Can you work these out from the model? Positions are in its coordinate system, mm. A direction names the side the tool comes from. Give positions to 0.01 mm unless a question says otherwise; leave off trailing zeros. Write each loop counter-clockwise with the first axis right and the second up, starting at its lowest first coordinate (ties: lowest second). Pieces come first, ordered by that corner, then holes.
from build123d import *

# Parameters (mm, degrees)
SKETCH1_W            = 52
SKETCH1_H            = 40
SKETCH1_R            = 2.75
BOSS_EXTRUDE10_DEPTH = 5
SKETCH1_21_R         = 2.75
BOSS_EXTRUDE13_DEPTH = 5
SKETCH1_22_R         = 2.12
CUT_EXTRUDE4_DEPTH   = 7
CHAMFER1_SIZE        = 1
SKETCH1_23_R         = 2.75
BOSS_EXTRUDE14_DEPTH = 5
SKETCH1_24_R         = 2.12
CUT_EXTRUDE6_DEPTH   = 5
SKETCH1_25_R         = 2.75
BOSS_EXTRUDE15_DEPTH = 5
SKETCH1_26_R         = 2.12
CUT_EXTRUDE7_DEPTH   = 18
SKETCH1_29_R         = 2.75
BOSS_EXTRUDE17_DEPTH = 5
SKETCH1_30_R         = 2.12
CUT_EXTRUDE9_DEPTH   = 14
CHAMFER3_SIZE        = 1
CHAMFER4_SIZE        = 1
CHAMFER5_SIZE        = 1
SKETCH5_W            = 104
SKETCH5_H            = 97.258090947
BOSS_EXTRUDE19_DEPTH = 8


with BuildPart() as part:
    # Sketch1 → Boss-Extrude10 (new body)
    with BuildSketch(Plane(origin=(0, 0, 0), x_dir=(1, 0, 0), z_dir=(0, 1, 0))):
        Rectangle(SKETCH1_W, SKETCH1_H)
        with Locations(Location((-20, 4, 0), (0, 0, 270))):
            Circle(SKETCH1_R, mode=Mode.SUBTRACT)
        with Locations(Location((20, 4, 0), (0, 0, 270))):
            Circle(SKETCH1_R, mode=Mode.SUBTRACT)
        with Locations(Location((-20, -12, 0), (0, 0, 270))):
            Circle(SKETCH1_R, mode=Mode.SUBTRACT)
        with Locations(Location((20, -12, 0), (0, 0, 270))):
            Circle(SKETCH1_R, mode=Mode.SUBTRACT)
    extrude(amount=BOSS_EXTRUDE10_DEPTH)

    # Sketch1_21 → Boss-Extrude13 (add)
    with BuildSketch(Plane(origin=(0, 0, 0), x_dir=(1, 0, 0), z_dir=(0, 1, 0))):
        with Locations((20, 4)):
            Circle(SKETCH1_21_R)
    extrude(amount=BOSS_EXTRUDE13_DEPTH)

    # Sketch1_22 → Cut-Extrude4 (cut)
    with BuildSketch(Plane(origin=(0, 0, 0), x_dir=(1, 0, 0), z_dir=(0, 1, 0))):
        with Locations(Location((20, 4, 0), (0, 0, 90))):
            Circle(SKETCH1_22_R)
    extrude(amount=CUT_EXTRUDE4_DEPTH, mode=Mode.SUBTRACT)

    # Chamfer1
    chamfer1_edges = [part.edges().sort_by_distance(p)[0] for p in [
        (20, 5, -1.88),
    ]]
    chamfer(chamfer1_edges, length=CHAMFER1_SIZE)

    # Sketch1_23 → Boss-Extrude14 (add)
    with BuildSketch(Plane(origin=(0, 0, 0), x_dir=(1, 0, 0), z_dir=(0, 1, 0))):
        with Locations((20, -12)):
            Circle(SKETCH1_23_R)
    extrude(amount=BOSS_EXTRUDE14_DEPTH)

    # Sketch1_24 → Cut-Extrude6 (cut)
    with BuildSketch(Plane(origin=(0, 0, 0), x_dir=(1, 0, 0), z_dir=(0, 1, 0))):
        with Locations(Location((20, -12, 0), (0, 0, 90))):
            Circle(SKETCH1_24_R)
    extrude(amount=CUT_EXTRUDE6_DEPTH, mode=Mode.SUBTRACT)

    # Sketch1_25 → Boss-Extrude15 (add)
    with BuildSketch(Plane(origin=(0, 0, 0), x_dir=(1, 0, 0), z_dir=(0, 1, 0))):
        with Locations((-20, -12)):
            Circle(SKETCH1_25_R)
    extrude(amount=BOSS_EXTRUDE15_DEPTH)

    # Sketch1_26 → Cut-Extrude7 (cut)
    with BuildSketch(Plane(origin=(0, 0, 0), x_dir=(1, 0, 0), z_dir=(0, 1, 0))):
        with Locations(Location((-20, -12, 0), (0, 0, 270))):
            Circle(SKETCH1_26_R)
    extrude(amount=CUT_EXTRUDE7_DEPTH, mode=Mode.SUBTRACT)

    # Sketch1_29 → Boss-Extrude17 (add)
    with BuildSketch(Plane(origin=(0, 0, 0), x_dir=(1, 0, 0), z_dir=(0, 1, 0))):
        with Locations((-20, 4)):
            Circle(SKETCH1_29_R)
    extrude(amount=BOSS_EXTRUDE17_DEPTH)

    # Sketch1_30 → Cut-Extrude9 (cut)
    with BuildSketch(Plane(origin=(0, 0, 0), x_dir=(1, 0, 0), z_dir=(0, 1, 0))):
        with Locations(Location((-20, 4, 0), (0, 0, 270))):
            Circle(SKETCH1_30_R)
    extrude(amount=CUT_EXTRUDE9_DEPTH, mode=Mode.SUBTRACT)

    # Chamfer3
    chamfer3_edges = [part.edges().sort_by_distance(p)[0] for p in [
        (-20, 5, -6.12),
    ]]
    chamfer(chamfer3_edges, length=CHAMFER3_SIZE)

    # Chamfer4
    chamfer4_edges = [part.edges().sort_by_distance(p)[0] for p in [
        (-20, 5, 9.88),
    ]]
    chamfer(chamfer4_edges, length=CHAMFER4_SIZE)

    # Chamfer5
    chamfer5_edges = [part.edges().sort_by_distance(p)[0] for p in [
        (20, 5, 14.12),
    ]]
    chamfer(chamfer5_edges, length=CHAMFER5_SIZE)

    # Sketch5 → Boss-Extrude19 (add)
    with BuildSketch(Plane(origin=(0, 0, 0), x_dir=(1, 0, 0), z_dir=(0, 1, 0))):
        with Locations((0, 16.370954527)):
            Rectangle(SKETCH5_W, SKETCH5_H)
        Polygon((26, -20), (-26, -20), (-26, 20), (0, 20), (26, 20), align=None, mode=Mode.SUBTRACT)
    extrude(amount=BOSS_EXTRUDE19_DEPTH)


solid = part.part
(1) If we mould it in two halves opening along Z, with no side actions, what happens to faces 3 (the face through (0, 6, 20)), 4 (the face through (-1, 8, -28)), 5 (the face through (-1, 4, 32.258))? For each: +Z half, -Z half, draft (parallel to the pull), parting line (faces both ways), or undercut.
Returned:
face 3: undercut
face 4: draft
face 5: +Z half
(2) Will these pins go through, and if not, where does the flat tip stop? P1, Ø2, axis at x = -19, z = 6.5, coming from the +Y side; P2, Ø5.5, axis at x = -20, z = 12, coming from the +Y side; P3, Ø5, axis at x = 20, z = -4, coming from the +Y side.
Returned:
P1: stops at y = 5
P2: stops at y = 4.63
P3: stops at y = 4.38
(3) Imagine slicing it at A-A, the plane x = -20. Write out the boundary of the cut face in (y, z).
Returned:
outline: (0, -65) - (8, -65) - (8, -20) - (5, -20) - (5, -7.12) - (4, -6.12) - (0, -6.12) - close; (0, -1.88) - (4, -1.88) - (5, -0.88) - (5, 8.88) - (4, 9.88) - (0, 9.88) - close; (0, 14.12) - (4, 14.12) - (5, 15.12) - (5, 20) - (8, 20) - (8, 32.26) - (0, 32.26) - close
(4) Imagine slicing it at C-C, the plane y = 6.25. Write out the boundary of the cut face in (x, z).
Returned:
outline: (-52, -65) - (52, -65) - (52, 32.26) - (-52, 32.26) - close; hole (-26, -20) - (26, -20) - (26, 20) - (-26, 20) - close
(5) For faces 1 (the face through (26, 6, 0)), 2 (the face through (-22.07, 1.97, -4.46)), which set-ups out of +Z, -Z, +X, -X, +Y, -Y let a thin tool reach every point of the face, with its end or its side?
Returned:
face 1: +Y
face 2: +Y, -Y
(6) If I drill on L1, parallel to X at y = 1.75, z = 12; L2, parallel to Z at x = 20, y = 2.4; L3, parallel to Z at x = -18, y = 6.25, over which ranges is the centre line in solid material (lowest first)?
Returned:
L1: x = -52 to -22.12, -17.88 to 17.88, 22.12 to 52
L2: z = -65 to -6.12, -1.88 to 9.88, 14.12 to 32.26
L3: z = -65 to -20, 20 to 32.26
(7) Imagine slicing it at B-B, the plane z = -4. Write out the boundary of the cut face in (x, y).
Returned:
outline: (-52, 0) - (-22.12, 0) - (-22.12, 4) - (-23.12, 5) - (-26, 5) - (-26, 8) - (-52, 8) - close; (-17.88, 0) - (17.88, 0) - (17.88, 4) - (16.88, 5) - (-16.88, 5) - (-17.88, 4) - close; (22.12, 0) - (52, 0) - (52, 8) - (26, 8) - (26, 5) - (23.12, 5) - (22.12, 4) - close
(8) Imagine slicing it at D-D, the plane x = -3. Write out the boundary of the cut face in (y, z), plus the area to 3 significant figures.
Returned:
outline: (0, -65) - (8, -65) - (8, -20) - (5, -20) - (5, 20) - (8, 20) - (8, 32.26) - (0, 32.26) - close
area: 658 mm2
